from build123d import *

# Parameters (mm, degrees)
ESQUISSE1_R      = 11
FOND_DEPTH       = 2
ESQUISSE2_R      = 16
CYLINDRE_1_DEPTH = 2
ESQUISSE3_R      = 12.5
CYLINDRE_2_DEPTH = 3
ESQUISSE4_R      = 16
CYLINDRE_3_DEPTH = 2
ESQUISSE5_R      = 12.5
CYLINDRE_4_DEPTH = 3.5
ESQUISSE6_R      = 16
CYLINDRE_5_DEPTH = 1
ESQUISSE7_R      = 10
CYLINDRE_6_DEPTH = 6
ESQUISSE8_R      = 6
CYLINDRE_7_DEPTH = 5
ESQUISSE9_R      = 4
CYLINDRE_8_DEPTH = 3
ESQUISSE12_R     = 6
CYLINDRE_9_DEPTH = 12
CHANFREIN1_SIZE  = 0.5
CHANFREIN2_SIZE  = 0.3
CHANFREIN3_SIZE  = 1


with BuildPart() as part:
    # Esquisse1 → fond (new body)
    with BuildSketch(Plane.XY):
        with Locations(Location((0, 0, 0), (0, 0, 180))):
            Circle(ESQUISSE1_R)
    extrude(amount=FOND_DEPTH)

    # Esquisse2 → cylindre 1 (add)
    with BuildSketch(Plane(origin=(0, 0, 0), x_dir=(-1, 0, 0), z_dir=(0, 0, -1))):
        Circle(ESQUISSE2_R)
    extrude(amount=CYLINDRE_1_DEPTH)

    # Esquisse3 → cylindre 2 (add)
    with BuildSketch(Plane(origin=(0, 0, -2), x_dir=(-1, 0, 0), z_dir=(0, 0, -1))):
        Circle(ESQUISSE3_R)
    extrude(amount=CYLINDRE_2_DEPTH)

    # Esquisse4 → cylindre 3 (add)
    with BuildSketch(Plane(origin=(0, 0, -5), x_dir=(-1, 0, 0), z_dir=(0, 0, -1))):
        Circle(ESQUISSE4_R)
    extrude(amount=CYLINDRE_3_DEPTH)

    # Esquisse5 → cylindre 4 (add)
    with BuildSketch(Plane(origin=(0, 0, -7), x_dir=(-1, 0, 0), z_dir=(0, 0, -1))):
        Circle(ESQUISSE5_R)
    extrude(amount=CYLINDRE_4_DEPTH)

    # Esquisse6 → cylindre 5 (add)
    with BuildSketch(Plane(origin=(0, 0, -10.5), x_dir=(-1, 0, 0), z_dir=(0, 0, -1))):
        Circle(ESQUISSE6_R)
    extrude(amount=CYLINDRE_5_DEPTH)

    # Esquisse7 → cylindre 6 (add)
    with BuildSketch(Plane(origin=(0, 0, -11.5), x_dir=(-1, 0, 0), z_dir=(0, 0, -1))):
        Circle(ESQUISSE7_R)
    extrude(amount=CYLINDRE_6_DEPTH)

    # Esquisse8 → cylindre 7 (add)
    with BuildSketch(Plane(origin=(0, 0, -17.5), x_dir=(-1, 0, 0), z_dir=(0, 0, -1))):
        with Locations(Location((0, 0, 0), (0, 0, 180))):
            Circle(ESQUISSE8_R)
    extrude(amount=CYLINDRE_7_DEPTH)

    # Esquisse9 → cylindre 8 (add)
    with BuildSketch(Plane(origin=(0, 0, -22.5), x_dir=(-1, 0, 0), z_dir=(0, 0, -1))):
        Circle(ESQUISSE9_R)
    extrude(amount=CYLINDRE_8_DEPTH)

    # Esquisse12 → cylindre 9 (add)
    with BuildSketch(Plane(origin=(0, 0, -25.5), x_dir=(-1, 0, 0), z_dir=(0, 0, -1))):
        with Locations(Location((0, 0, 0), (0, 0, 180))):
            Circle(ESQUISSE12_R)
    extrude(amount=CYLINDRE_9_DEPTH)

    # gorge: sweep along a path in Esquisse16
    with BuildLine(Plane.XY.offset(-32.5)) as gorge_path:
        CenterArc((0, 0), 2, 0, 360)
    # Esquisse13 → gorge (sweep, cut)
    with BuildSketch(Plane(origin=(0, 0, 0), x_dir=(1, 0, 0), z_dir=(0, 1, 0))):
        with BuildLine():
            Line((-10.48576902, 34.5), (-4, 34.5))
            ThreePointArc((-4, 34.5), (-2, 32.5), (-4, 30.5))
            Line((-4, 30.5), (-10.48576902, 30.5))
            Line((-10.48576902, 30.5), (-10.48576902, 34.5))
        make_face()
    sweep(path=gorge_path.line, mode=Mode.SUBTRACT)

    # Chanfrein1
    chanfrein1_edges = [part.edges().sort_by_distance(p)[0] for p in [
        (-6, 0, -25.5),
        (-5.999999999, -2e-09, -30.5),
        (-6, 0, -22.5),
        (-5.999999999, -2e-09, -34.5),
        (-6, 0, -37.5),
        (10, 0, -17.5),
        (12.5, 0, -7),
        (16, 0, -7),
        (16, 0, -5),
    ]]
    chamfer(chanfrein1_edges, length=CHANFREIN1_SIZE)

    # Chanfrein2
    chanfrein2_edges = [part.edges().sort_by_distance(p)[0] for p in [
        (16, 0, -11.5),
        (16, 0, -10.5),
    ]]
    chamfer(chanfrein2_edges, length=CHANFREIN2_SIZE)

    # Chanfrein3
    chanfrein3_edges = [part.edges().sort_by_distance(p)[0] for p in [
        (16, 0, 0),
    ]]
    chamfer(chanfrein3_edges, length=CHANFREIN3_SIZE)


solid = part.part
Read the model definition and answer for the solid it produces. Units are mm, in the model's axes. A direction names the side the tool comes from. Round coordinates to 2 decimals unless told otherwise and drop trailing zeros. Order: outer loops, then holes, each group sorted by start corner. A loop starts at its lowest first (then second) coordinate and runs counter-clockwise, first axis right, second up.
1) The mould has two halves that part along Z. Classify faces 1 (the face through (-4, 2, -25.5)), 2 (the face through (0, 0, -37.5)), 3 (the face through (0, 0, 2)), 4 (the face through (3.47, -15.62, -5.99)): released by +Z, released by -Z, zero draft, split by the parting line, or undercut.
2) The part is cut by section A-A on z = -29. Write down the section's boundary in (x, y), plus the area to 3 significant figures.
3) Straight lines are drawn through the part: L1, parallel to Z at x = -3, y = 4.5; L2, parallel to Z at x = 11, y = -8.5; L3, parallel to Z at x = -4, y = -5. For each, find the intervals that lie inside material, in ascending order.
4) Flat-ended cylindrical pins translate along their axes: pin 1 (1 mm diameter, centred on y = -5.5, z = -16.5, fed in from +X); pin 2 (5 mm diameter, centred on x = -3, y = 11, fed in from -Z); pin 3 (3 mm diameter, centred on y = 1, z = -14.5, fed in from -X). Find the tip coordinate at first contact, or state that the pin passes through.
5) The part is cut by section D-D on z = -33.5. Write down the section's boundary in (x, y).
6) The part is cut by section B-B on x = -13.5. Give the number of separate pieces and of enclosed holes in the cut face, plus the area to 3 significant figures.
7) For faces 5 (the face through (5.723, -1.802, -35.986)), 6 (the face through (0.867, -3.905, -23.979)), 7 (the face through (2.38, 10.74, 0.99)), determine the directions among +Z, -Z, +X, -X, +Y, -Y from which every point of the face is accessible in a straight line to the end or side of a thin tool.
Resolved:
1. face 1: undercut
1. face 2: released by -Z
1. face 3: released by +Z
1. face 4: zero draft
2. outline: circle Ø12 at (0, 0)
2. area: 113 mm2
3. L1: z = -37.5 to -34.5, -30.5 to -25.5, -22.5 to 2
3. L2: z = -11.5 to -10.5, -7 to -5, -2 to 0
3. L3: z = -17.5 to 2
4. pin 1: stops at x = 8.66
4. pin 2: stops at z = -17.5
4. pin 3: stops at x = -10
5. outline: circle Ø4.54 at (0, 0)
6. separate pieces: 3
6. enclosed holes: 0
6. area: 82.6 mm2
7. face 5: -Z
7. face 6: none
7. face 7: +Z
